Design review of the part built by this model. Coordinates are the model's own, in mm. Give positions to 0.01 mm unless a question says otherwise; leave off trailing zeros. Order: outer loops, then holes, each group sorted by start corner. A loop starts at its lowest first (then second) coordinate and runs counter-clockwise, first axis right, second up. Notation, with made-up numbers: (-3.5, -8) -> (27.5, -8) arc R21 ccw to (27.5, -4) -> close; hole circle Ø8 at (25.25, 25). An arc over 180 degrees is marked (long way). Return JSON: item names as keys, results as strings.
```python
from build123d import *

# Parameters (mm, degrees)
SKETCH1_W           = 137.16
SKETCH1_H           = 106.68
BOSS_EXTRUDE1_DEPTH = 1
SKETCH4_W           = 2.54
SKETCH4_H           = 2.54
BOSS_EXTRUDE2_DEPTH = 2.54
SKETCH5_W           = 69.85
SKETCH5_H           = 50.8
CUT_EXTRUDE1_DEPTH  = 2.54


with BuildPart() as part:
    # Sketch1 → Boss-Extrude1 (new body)
    with BuildSketch(Plane.XY):
        Rectangle(SKETCH1_W, SKETCH1_H)
    extrude(amount=BOSS_EXTRUDE1_DEPTH)

    # Sketch4 → Boss-Extrude2 (add)
    with BuildSketch(Plane.XY.offset(1)):
        with Locations((-48.26, 33.02)):
            Rectangle(SKETCH4_W, SKETCH4_H)
        with Locations((48.26, 33.02)):
            Rectangle(SKETCH4_W, SKETCH4_H)
        with Locations((48.26, -33.02)):
            Rectangle(SKETCH4_W, SKETCH4_H)
        with Locations((-48.26, -33.02)):
            Rectangle(SKETCH4_W, SKETCH4_H)
    extrude(amount=BOSS_EXTRUDE2_DEPTH)

    # Sketch5 → Cut-Extrude1 (cut)
    with BuildSketch(Plane.XY.offset(1)):
        Rectangle(SKETCH5_W, SKETCH5_H)
    extrude(amount=-CUT_EXTRUDE1_DEPTH, mode=Mode.SUBTRACT)


solid = part.part
```
Item 1: For pin 1 (0.8 mm diameter, centred on y = -33, z = 2, fed in from -X); pin 2 (2 mm diameter, centred on x = -48.5, z = 2.5, fed in from +Y); pin 3 (0.8 mm diameter, centred on y = -33, z = 2.5, fed in from +X); pin 4 (3 mm diameter, centred on x = 17, y = 22.5, fed in from +Z), all flat-tipped, find the tip position at first contact; note any pin that passes through.
Result set:
{"pin 1": "stops at x = -49.53", "pin 2": "stops at y = 34.29", "pin 3": "stops at x = 49.53", "pin 4": "passes through"}
Item 2: Wall thickness on L1, parallel to Y at x = 7, z = 0.5; L2, parallel to X at y = 24.5, z = 0.4 (3 decimals); L3, parallel to Z at x = -8, y = 43.5: over which ranges is each line inside the solid? List them lowest first. Write a range as [from, to].
Result set:
{"L1": "y = [-53.34, -25.4], [25.4, 53.34]", "L2": "x = [-68.58, -34.925], [34.925, 68.58]", "L3": "z = [0, 1]"}
Item 3: Add section D-D (x = 51). Give the boundary of the cut face in (y, z).
Result set:
{"outline": "(-53.34, 0) -> (53.34, 0) -> (53.34, 1) -> (-53.34, 1) -> close"}
Item 4: Add section B-B (z = 2.8). Give the boundary of the cut face in (x, y).
Result set:
{"outline": "(-49.53, -34.29) -> (-46.99, -34.29) -> (-46.99, -31.75) -> (-49.53, -31.75) -> close; (-49.53, 31.75) -> (-46.99, 31.75) -> (-46.99, 34.29) -> (-49.53, 34.29) -> close; (46.99, -34.29) -> (49.53, -34.29) -> (49.53, -31.75) -> (46.99, -31.75) -> close; (46.99, 31.75) -> (49.53, 31.75) -> (49.53, 34.29) -> (46.99, 34.29) -> close"}
Item 5: Add section C-C (y = 19.5). Give the boundary of the cut face in (x, z) (3 decimals), plus the area to 3 significant figures.
Result set:
{"outline": "(-68.58, 0) -> (-34.925, 0) -> (-34.925, 1) -> (-68.58, 1) -> close; (34.925, 0) -> (68.58, 0) -> (68.58, 1) -> (34.925, 1) -> close", "area": "67.3 mm^2"}
Item 6: Add section A-A (x = 29.5). Give the boundary of the cut face in (y, z).
Result set:
{"outline": "(-53.34, 0) -> (-25.4, 0) -> (-25.4, 1) -> (-53.34, 1) -> close; (25.4, 0) -> (53.34, 0) -> (53.34, 1) -> (25.4, 1) -> close"}
